Could you check a few things on this drawing? It's one solid part, dimensions in mm from its lowest x, y, z. A direction names the side the tool comes from. Give positions to 0.01 mm unless a question says otherwise; leave off trailing zeros. Loops run counter-clockwise (first coordinate to the right, second up) from the corner with the lowest first, then second, coordinate; pieces in that order, holes last.
Q1. I need wall thicknesses on probe 1 along Y at (x, z) = (37, 2) (1 decimal); probe 2 along Y at (x, z) = (10, 13.5) (1 decimal); probe 3 along X at (y, z) = (7, 4) (1 decimal). Which ranges of each line are inside material? Lowest first, please.
Q2. Suppose I cut it at C-C (x = 37.5). List the corners of the cut face in (y, z) for me, and give its area (3 significant figures).
Q3. Thinking about a two-plate mould opening in Y: for the marked faces 1, 2, 3 and 4, which applies, pulls with the +Y half, pulls with the -Y half, needs draft (parallel to the pull), parting line crosses it, or undercut?
Q4. Suppose I cut it at D-D (y = 10). List the corners of the cut face in (x, z) for me.
Q5. Suppose I cut it at B-B (y = 32). List the corners of the cut face in (x, z) for me.
Q6. For the marked faces 5, 6 and 7, which set-ups out of +Z, -Z, +X, -X, +Y, -Y let a thin tool reach every point of the face, with its end or its side?
Q7. Suppose I cut it at A-A (z = 11.5). List the corners of the cut face in (x, y) for me (1 decimal), and give its area (3 significant figures).
Q8. I'm going to push flat-ended pins straight in: P1, Ø2, axis at x = 24.5, z = 12, coming from the -Y side; P2, Ø10, axis at y = 15, z = 6, coming from the -X side; P3, Ø2.5, axis at y = 4.5, z = 16, coming from the -X side; P4, Ø5, axis at x = 24, y = 39, coming from the -Z side. Where does each tip first touch, or does it pass through?
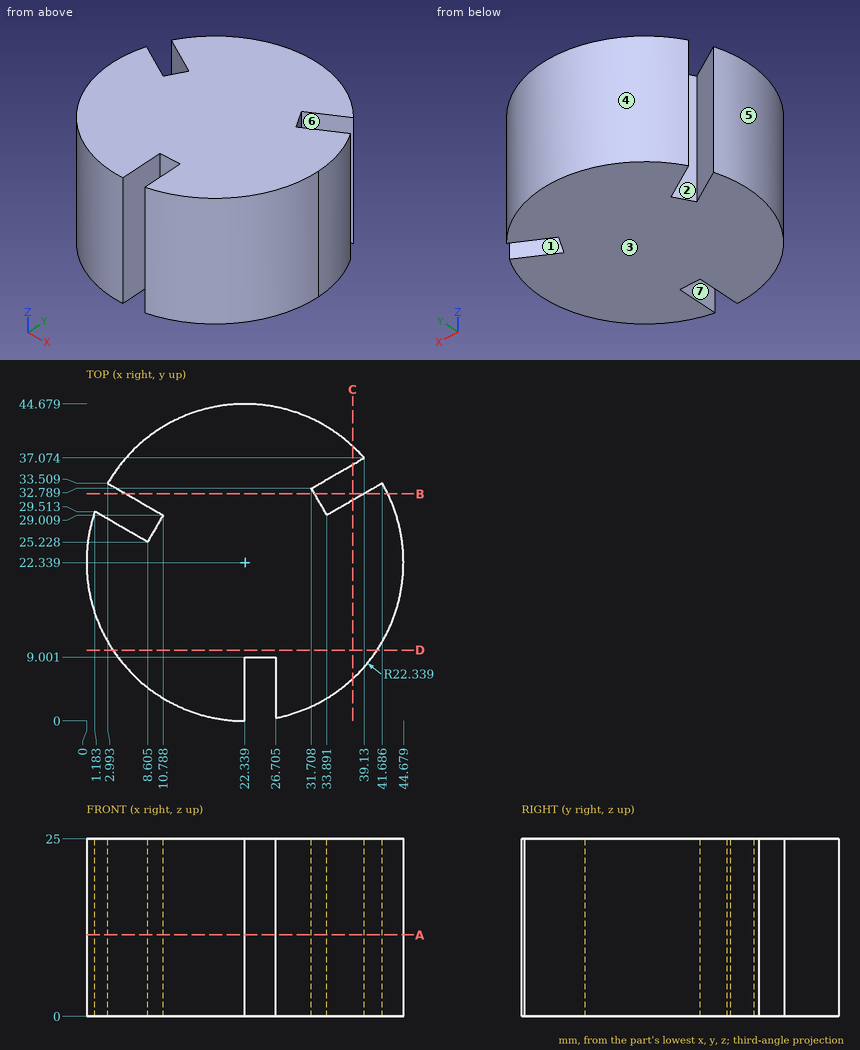
Solutions:
1. probe 1: y = 5.5 to 30.8, 35.8 to 39.2
1. probe 2: y = 3.7 to 27.6, 29.5 to 41
1. probe 3: x = 6.1 to 22.3, 26.7 to 38.6
2. outline: (5.93, 0) - (31.09, 0) - (31.09, 25) - (5.93, 25) - close; (36.13, 0) - (38.75, 0) - (38.75, 25) - (36.13, 25) - close
2. area: 694 mm2
3. face 1: undercut
3. face 2: undercut
3. face 3: needs draft
3. face 4: pulls with the +Y half
4. outline: (3.72, 0) - (40.96, 0) - (40.96, 25) - (3.72, 25) - close
5. outline: (5.61, 0) - (32.16, 0) - (32.16, 25) - (5.61, 25) - close; (39.07, 0) - (42.48, 0) - (42.48, 25) - (39.07, 25) - close
6. face 5: +Z, -Z, -X
6. face 6: +Z, -Z
6. face 7: +Z, -Z, -Y
7. outline: (1.2, 29.5) arc R22.3 ccw to (22.3, 0) - (22.3, 9) - (26.7, 9) - (26.7, 0.4) arc R22.3 ccw to (41.7, 33.5) - (33.9, 29) - (31.7, 32.8) - (39.1, 37.1) arc R22.3 ccw to (3, 33.5) - (10.8, 29) - (8.6, 25.2) - close
7. area: 1,450 mm2
8. P1: stops at y = 9
8. P2: stops at x = 0.12
8. P3: stops at x = 7.38
8. P4: stops at z = 0
